Build history of the part. All positions in model axes, mm. A direction names the side the tool comes from. Round coordinates to 2 decimals unless told otherwise and drop trailing zeros. Loops run counter-clockwise (first coordinate to the right, second up) from the corner with the lowest first, then second, coordinate; pieces in that order, holes last. Notation, with made-up numbers: M 70.25,-31 L 102.25,-31 A30 ccw 102.25,-7 Z; hole C -35.75,65 d5. An arc over 180 degrees is marked long. One line per item, written item: value.
```python
from build123d import *

# Parameters (mm, degrees)
F0_W     = 750
F0_H     = 1100
F1_DEPTH = 10
F2_W     = 750
F2_H     = 400
F3_DEPTH = 10
F4_W     = 300
F4_H     = 400
F5_DEPTH = 25
F6_R     = 60


with BuildPart() as f1:
    # F0 (on Top) → F1 (new body)
    with BuildSketch(Plane.XY):
        with Locations((-375, 550)):
            Rectangle(F0_W, F0_H)
    extrude(amount=F1_DEPTH)

    # F2 (on face) → F3 (join)
    with BuildSketch(Plane.XY.offset(10)):
        with Locations((-375, 1300)):
            Rectangle(F2_W, F2_H)
    extrude(amount=-F3_DEPTH)

    # F4 (on face) → F5 (cut)
    with BuildSketch(Plane.XY.offset(10)):
        with Locations((-250, 800)):
            Rectangle(F4_W, F4_H)
    extrude(amount=-F5_DEPTH, mode=Mode.SUBTRACT)

    # F6
    f6_edges = [f1.edges().sort_by_distance(p)[0] for p in [
        (-400, 1000, 5),
        (-400, 600, 5),
        (-100, 1000, 5),
        (-100, 600, 5),
    ]]
    fillet(f6_edges, radius=F6_R)


solid = f1.part
```
Item 1: Pull direction X, two halves, no side cores. Call faces 3 (the face through (-118.04, 617.11, 4.93)), 4 (the face through (-464, 760, 0)): pulls with the +X half, pulls with the -X half, needs draft (parallel to the pull), parting line crosses it, or undercut.
Check values:
face 3: undercut
face 4: needs draft
Item 2: Slice it at A-A, the plane x = -217.5. Give the cut face in (y, z), and give its area (3 significant figures).
Check values:
outline: M 0,0 L 600,0 L 600,10 L 0,10 Z; M 1000,0 L 1500,0 L 1500,10 L 1000,10 Z
area: 11,000 mm2
Item 3: Which spindle directions (+Z, -Z, +X, -X, +Y, -Y) get a long thin tool onto all of the face, cutting with end or side? Do faces 1 (the face through (-464, 760, 10)), 2 (the face through (-381.96, 617.11, 4.93)). Say none if no direction does.
Check values:
face 1: +Z, +X, -X, +Y, -Y
face 2: +Z, -Z
Item 4: Slice it at C-C, the plane z = 6.25. Give the cut face in (x, y), and give its area (3 significant figures).
Check values:
outline: M -750,0 L 0,0 L 0,1500 L -750,1500 Z; hole M -400,660 A60 ccw -340,600 L -160,600 A60 ccw -100,660 L -100,940 A60 ccw -160,1000 L -340,1000 A60 ccw -400,940 Z
area: 1,010,000 mm2
Item 5: Wall check: line 1 along X through (y, z) = (914.5, 6.5); line 2 along Y through (x, z) = (-186, 5.5); line 3 along Y through (x, z) = (-370.5, 9). Give the ranges that are in metal, low to high.
Check values:
line 1: x = -750 to -400, -100 to 0
line 2: y = 0 to 600, 1000 to 1500
line 3: y = 0 to 608.33, 991.67 to 1500
Item 6: Slice it at B-B, the plane y = 899. Give the cut face in (x, z), and give its area (3 significant figures).
Check values:
outline: M -750,0 L -400,0 L -400,10 L -750,10 Z; M -100,0 L 0,0 L 0,10 L -100,10 Z
area: 4,500 mm2
